Check sheet for the modelled part. Datum: model origin and axes. Units: mm. Face numbers are marked on the shaded views. A direction names the side the tool comes from. Give positions to 0.01 mm unless a question says otherwise; leave off trailing zeros. Order: outer loops, then holes, each group sorted by start corner. A loop starts at its lowest first (then second) coordinate and runs counter-clockwise, first axis right, second up.
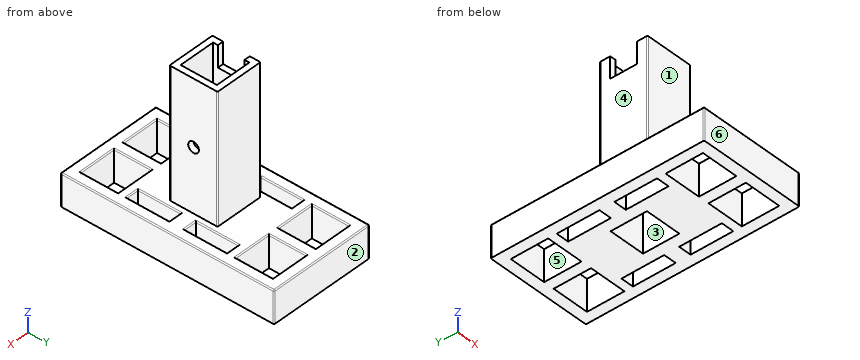
Solid Edge part; units mm, degrees
sketch "Sketch1" plane through (0, 0, 0) normal (0, 0, 1) x (1, 0, 0)
  line L0 (100, 0) -> (100, 200)
  line L1 (100, 200) -> (0, 200)
  line L2 (0, 200) -> (0, 0)
  line L3 (0, 0) -> (100, 0)
extrude "Protrusion1" add sketch "Sketch1" along normal blind 30
sketch "Sketch2" plane through (50, 100, 30) normal (0, 0, 1) x (0, 1, 0)
  line L0 (-55, 40) -> (-90, 40)
  line L1 (-90, 40) -> (-90, 5)
  line L2 (-90, 5) -> (-55, 5)
  line L3 (-55, 5) -> (-55, 40)
  line L4 (-7, 40) -> (-47, 40)
  line L5 (-47, 40) -> (-47, 28)
  line L6 (-47, 28) -> (-7, 28)
  line L7 (-7, 28) -> (-7, 40)
  line L8 (7, 40) -> (47, 40)
  line L9 (47, 40) -> (47, 28)
  line L10 (47, 28) -> (7, 28)
  line L11 (7, 28) -> (7, 40)
  line L12 (55, 40) -> (90, 40)
  line L13 (90, 40) -> (90, 5)
  line L14 (90, 5) -> (55, 5)
  line L15 (55, 5) -> (55, 40)
  line L16 (-55, -40) -> (-55, -5)
  line L17 (-55, -5) -> (-90, -5)
  line L18 (-90, -5) -> (-90, -40)
  line L19 (-90, -40) -> (-55, -40)
  line L20 (-7, -28) -> (-47, -28)
  line L21 (-47, -28) -> (-47, -40)
  line L22 (-47, -40) -> (-7, -40)
  line L23 (-7, -40) -> (-7, -28)
  line L24 (7, -28) -> (47, -28)
  line L25 (47, -28) -> (47, -40)
  line L26 (47, -40) -> (7, -40)
  line L27 (7, -40) -> (7, -28)
  line L28 (55, -40) -> (55, -5)
  line L29 (55, -5) -> (90, -5)
  line L30 (90, -5) -> (90, -40)
  line L31 (90, -40) -> (55, -40)
  line L32 (17, -17) -> (17, 17)
  line L33 (17, 17) -> (-17, 17)
  line L34 (-17, 17) -> (-17, -17)
  line L35 (-17, -17) -> (17, -17)
extrude "Cutout1" cut sketch "Sketch2" against normal up to next
sketch "Sketch3" plane through (50, 100, 30) normal (0, 0, 1) x (0, 1, 0)
  line L0 (22.5, 22.5) -> (-22.5, 22.5)
  line L1 (-22.5, 22.5) -> (-22.5, -22.5)
  line L2 (-22.5, -22.5) -> (22.5, -22.5)
  line L3 (22.5, -22.5) -> (22.5, 22.5)
  line L4 (17, 17) -> (-17, 17)
  line L5 (-17, 17) -> (-17, -17)
  line L6 (-17, -17) -> (17, -17)
  line L7 (17, -17) -> (17, 17)
extrude "ExtrudedProtrusion_2" add sketch "Sketch3" along normal blind 120
sketch "Sketch4" plane through (72.5, 100, 105) normal (1, 0, 0) x (0, 1, 0)
  circle A0 centre (0, -16.1) radius 5
extrude "Cutout2" cut sketch "Sketch4" against normal up to next
fillet "Round_1" radius 1 44 edges at (100, 100, 30) (50, 0, 30) (50, 200, 30) (0, 100, 30) (0, 200, 15) (100, 200, 15) (100, 0, 15) (0, 0, 15) (72.5, 77.5, 90) (72.5, 122.5, 90) (27.5, 77.5, 90) (27.5, 122.5, 90) (10, 27.5, 30) (27.5, 10, 30) (27.5, 45, 30) (45, 27.5, 30) (55, 27.5, 30) (72.5, 10, 30) (72.5, 45, 30) (90, 27.5, 30) (78, 73, 30) (84, 53, 30) (90, 73, 30) (84, 93, 30) (78, 127, 30) (84, 107, 30) (90, 127, 30) (84, 147, 30) (72.5, 155, 30) (55, 172.5, 30) (72.5, 190, 30) (90, 172.5, 30) (10, 172.5, 30) (27.5, 190, 30) (27.5, 155, 30) (45, 172.5, 30) (10, 73, 30) (16, 53, 30) (22, 73, 30) (16, 93, 30) (16, 147, 30) (22, 127, 30) (10, 127, 30) (16, 107, 30)
sketch "Sketch5" plane through (27.5, 100, 105) normal (-1, 0, 0) x (0, -1, 0)
  line L0 (-12.5, 45) -> (-12.5, 25)
  line L1 (-12.5, 25) -> (12.5, 25)
  line L2 (12.5, 25) -> (12.5, 45)
  line L3 (12.5, 45) -> (-12.5, 45)
extrude "Cutout3" cut sketch "Sketch5" against normal up to next
Q1. Draft check along Y on the marked faces 1, 2 and 3. Enter one of: pulls with the +Y half, pulls with the -Y half, needs draft (parallel to the pull), parting line crosses it, or undercut.
Q2. Sectioned sample at B-B, the plane y = 100. Record the cut outline in (x, z), plus the area to 3 significant figures.
Q3. Sectioned sample at D-D, the plane z = 98. Record the cut outline in (x, y), plus the area to 3 significant figures.
Q4. Material ranges on line 1 (X direction, y = 37, z = 23.5); line 2 (Y direction, x = 44.5, z = 92); line 3 (Z direction, x = 69.4, y = 100), recorded low to high.
Q5. Tool access check on the marked faces 4, 5 and 6. Record the directions out of +Z, -Z, +X, -X, +Y, -Y that give a thin tool (end or side, any length) a straight path to the whole face; none if there is none.
Q6. Sectioned sample at A-A, the plane x = 18. Count the separate pieces of the cut face and the enclosed holes in it, plus the area to 3 significant figures.
Q7. Sectioned sample at C-C, the plane x = 60. Record the cut outline in (y, z), plus the area to 3 significant figures.
Q8. Go/stop test with flat-tipped pins: P1, Ø14.5, axis at x = 30, z = 13, coming from the -Y side; P2, Ø8, axis at x = 47, z = 117, coming from the +Y side; P3, Ø13, axis at y = 90, z = 100, coming from the -X side; P4, Ø10, axis at x = 40, y = 68, coming from the +Z side. Record where each tip stops, or that it passes through.
Filled in:
1. face 1: pulls with the -Y half
1. face 2: pulls with the +Y half
1. face 3: undercut
2. outline: (0, 0) - (33, 0) - (33, 130) - (27.5, 130) - (27.5, 30) - (1, 30) arc R1 ccw to (0, 29) - close; (67, 0) - (100, 0) - (100, 29) arc R1 ccw to (99, 30) - (72.5, 30) - (72.5, 83.9) - (67, 83.9) - close; (67, 93.9) - (72.5, 93.9) - (72.5, 150) - (67, 150) - close
2. area: 3,130 mm2
3. outline: (27.5, 78.5) arc R1 ccw to (28.5, 77.5) - (71.5, 77.5) arc R1 ccw to (72.5, 78.5) - (72.5, 121.5) arc R1 ccw to (71.5, 122.5) - (28.5, 122.5) arc R1 ccw to (27.5, 121.5) - close; hole (33, 83) - (67, 83) - (67, 117) - (33, 117) - close
3. area: 868 mm2
4. line 1: x = 0 to 10, 45 to 55, 90 to 100
4. line 2: y = 77.5 to 83, 117 to 122.5
4. line 3: z = 0 to 83.9, 93.9 to 150
5. face 4: +Z, -X, +Y, -Y
5. face 5: +Z, -Z
5. face 6: +Z, -Z, +X, -X, -Y
6. separate pieces: 5
6. enclosed holes: 0
6. area: 1,500 mm2
7. outline: (0, 0) - (10, 0) - (10, 29) arc R1 ccw to (9, 30) - (1, 30) arc R1 ccw to (0, 29) - close; (45, 0) - (83, 0) - (83, 150) - (77.5, 150) - (77.5, 30) - (46, 30) arc R1 ccw to (45, 29) - close; (117, 0) - (155, 0) - (155, 29) arc R1 ccw to (154, 30) - (122.5, 30) - (122.5, 150) - (117, 150) - close; (190, 0) - (200, 0) - (200, 29) arc R1 ccw to (199, 30) - (191, 30) arc R1 ccw to (190, 29) - close
7. area: 4,200 mm2
8. P1: stops at y = 0
8. P2: stops at y = 122.5
8. P3: stops at x = 27.5
8. P4: stops at z = 30
